```python
from build123d import *

# Parameters (mm, degrees)
F0_R     = 7.5
F0_R_2   = 3.125
F1_DEPTH = 10
F2_DEPTH = 4


with BuildPart() as f1:
    # F0 (on Top) → F1 (new body)
    with BuildSketch(Plane.XY):
        Circle(F0_R)
        Polygon((3.031089, 5.25), (6.062178, 0), (3.031089, -5.25), (-3.031089, -5.25), (-6.062178, 0), (-3.031089, 5.25), align=None, mode=Mode.SUBTRACT)
        Polygon((3.031089, -5.25), (6.062178, 0), (3.031089, 5.25), (-3.031089, 5.25), (-6.062178, 0), (-3.031089, -5.25), align=None)
        Circle(F0_R_2, mode=Mode.SUBTRACT)
    extrude(amount=F1_DEPTH)

    # F0 (on Top) → F2 (cut)
    with BuildSketch(Plane.XY):
        Polygon((3.031089, -5.25), (6.062178, 0), (3.031089, 5.25), (-3.031089, 5.25), (-6.062178, 0), (-3.031089, -5.25), align=None)
        Circle(F0_R_2, mode=Mode.SUBTRACT)
    extrude(amount=F2_DEPTH, mode=Mode.SUBTRACT)


solid = f1.part
```
Input: part model. Units: mm. Frame: model coordinates. A direction names the side the tool comes from. Coordinates: 2 decimals unless noted, no trailing zeros. Loops run counter-clockwise (first coordinate to the right, second up) from the corner with the lowest first, then second, coordinate; pieces in that order, holes last.
Q1. Contact query for flat-ended pins moving along their axis: pin 1 (4 mm diameter, centred on y = -2.5, z = 3.5, fed in from +X); pin 2 (3 mm diameter, centred on x = -5, z = 1.5, fed in from +Y); pin 3 (1.5 mm diameter, centred on x = 2.5, y = 0, fed in from -Z). Output: stop coordinate, or through.
Results are:
pin 1: stops at x = 7.48
pin 2: stops at y = 6.63
pin 3: stops at z = 4
Q2. Mould query, pull axis Y, two halves, no side actions, for faces 3 (the flat face through (3, 2, 4)), 4 (the flat face through (4.568, 2.588, 1.972)), 5 (the cylindrical face through (-7.493, 0.33, 4.93)), 6 (the flat face through (2, -3, 10)). Classes: +Y half, -Y half, draft (parallel to the pull), parting line (faces both ways), or undercut.
Results are:
face 3: undercut
face 4: undercut
face 5: parting line
face 6: draft
Q3. Section A-A, the plane x = 0. Return the cut outline in (y, z) (3 decimals).
Results are:
outline: (-7.5, 0) - (-5.25, 0) - (-5.25, 4) - (-3.125, 4) - (-3.125, 10) - (-7.5, 10) - close; (3.125, 4) - (5.25, 4) - (5.25, 0) - (7.5, 0) - (7.5, 10) - (3.125, 10) - close
Q4. Set-up query: faces 1 (the flat face through (-4.568, -2.588, 1.972)), 2 (the cylindrical face through (2.98, 0.94, 6.96)). Return all of +Z, -Z, +X, -X, +Y, -Y with unobstructed straight access to the full face (end or side cutting, diameter ignored); none if empty.
Results are:
face 1: -Z
face 2: +Z, -Z
Q5. Line query: line 1 along Y through (x, z) = (0, 5.85) (3 decimals); line 2 along X through (y, z) = (-1, 4.25); line 3 along Y through (x, z) = (-2.75, 3.75). Output: solid intervals per line, ascending.
Results are:
line 1: y = -7.5 to -3.125, 3.125 to 7.5
line 2: x = -7.43 to -2.96, 2.96 to 7.43
line 3: y = -6.98 to -5.25, 5.25 to 6.98
Q6. Section C-C, the plane y = 0.75. Return the cut outline in (x, z).
Results are:
outline: (-7.46, 0) - (-5.63, 0) - (-5.63, 4) - (-3.03, 4) - (-3.03, 10) - (-7.46, 10) - close; (3.03, 4) - (5.63, 4) - (5.63, 0) - (7.46, 0) - (7.46, 10) - (3.03, 10) - close
Q7. Section D-D, the plane y = 5. Return the cut outline in (x, z), and give its area (3 significant figures).
Results are:
outline: (-5.59, 0) - (-3.18, 0) - (-3.18, 4) - (3.18, 4) - (3.18, 0) - (5.59, 0) - (5.59, 10) - (-5.59, 10) - close
area: 86.4 mm2
Q8. Section B-B, the plane z = 2. Return the cut outline in (x, y).
Results are:
outline: circle Ø15 at (0, 0); hole (-6.06, 0) - (-3.03, -5.25) - (3.03, -5.25) - (6.06, 0) - (3.03, 5.25) - (-3.03, 5.25) - close
